from build123d import *

# Parameters (mm, degrees)
SKETCH2_R           = 2.55
SKETCH2_R_2         = 1.75
SKETCH2_R_3         = 11.5
SKETCH2_R_4         = 2.25
SKETCH2_R_5         = 2.6
BOSS_EXTRUDE1_DEPTH = 3


with BuildPart() as part:
    # Sketch2 → Boss-Extrude1 (new body)
    with BuildSketch(Plane(origin=(0, 0, 0), x_dir=(1, 0, 0), z_dir=(0, 1, 0))):
        with BuildLine():
            Line((0, -16.785), (0, 16.785))
            ThreePointArc((0, 16.785), (0.990365412, 21.123949711), (3.76529692, 24.603470279))
            Line((3.76529692, 24.603470279), (30.285548105, 45.751583128))
            ThreePointArc((30.285548105, 45.751583128), (42.973931455, 47.180980298), (49.767191801, 36.369418793))
            Line((49.767191801, 36.369418793), (49.767191801, 22.869418793))
            ThreePointArc((49.767191801, 22.869418793), (53.281910427, 14.384137419), (61.767191801, 10.869418793))
            Line((61.767191801, 10.869418793), (100.597191801, 10.869418793))
            ThreePointArc((100.597191801, 10.869418793), (105.807473987, 9.207876366), (109.093955082, 4.836743136))
            ThreePointArc((109.093955082, 4.836743136), (109.021446628, -3.277934075), (103.801176734, -9.490986945))
            Line((103.801176734, -9.490986945), (92.738459269, -15.929642261))
            ThreePointArc((92.738459269, -15.929642261), (89.099691246, -19.587512883), (87.768658735, -24.572390281))
            Line((87.768658735, -24.572390281), (87.768658735, -36.122390281))
            ThreePointArc((87.768658735, -36.122390281), (84.839726547, -43.193458093), (77.768658735, -46.122390281))
            Line((77.768658735, -46.122390281), (37.768658735, -46.122390281))
            ThreePointArc((37.768658735, -46.122390281), (34.279940347, -45.58043956), (31.120041688, -44.005667499))
            Line((31.120041688, -44.005667499), (4.218593872, -24.944371494))
            ThreePointArc((4.218593872, -24.944371494), (1.117037057, -21.377708281), (0, -16.785))
        make_face()
        with Locations(Location((37.767191801, 36.369418793, 0), (0, 0, 270))):
            Circle(SKETCH2_R, mode=Mode.SUBTRACT)
        with Locations(Location((37.767191801, 16.369418793, 0), (0, 0, 270))):
            Circle(SKETCH2_R_2, mode=Mode.SUBTRACT)
        with Locations(Location((22.26, 0.877609719, 0), (0, 0, 270))):
            Circle(SKETCH2_R_3, mode=Mode.SUBTRACT)
        with Locations(Location((37.767191801, -14.630581207, 0), (0, 0, 270))):
            Circle(SKETCH2_R_2, mode=Mode.SUBTRACT)
        with Locations(Location((6.767191801, -14.630581207, 0), (0, 0, 270))):
            Circle(SKETCH2_R_2, mode=Mode.SUBTRACT)
        with Locations(Location((6.767191801, 16.369418793, 0), (0, 0, 270))):
            Circle(SKETCH2_R_2, mode=Mode.SUBTRACT)
        with Locations(Location((52.26, 0.877609719, 0), (0, 0, 270))):
            Circle(SKETCH2_R_4, mode=Mode.SUBTRACT)
        with Locations(Location((78.26, 0.877609719, 0), (0, 0, 270))):
            Circle(SKETCH2_R_4, mode=Mode.SUBTRACT)
        with Locations(Location((97.86, 0.877609719, 0), (0, 0, 270))):
            Circle(SKETCH2_R_5, mode=Mode.SUBTRACT)
        with Locations(Location((37.767191801, -34.630581207, 0), (0, 0, 270))):
            Circle(SKETCH2_R, mode=Mode.SUBTRACT)
    extrude(amount=BOSS_EXTRUDE1_DEPTH)


solid = part.part
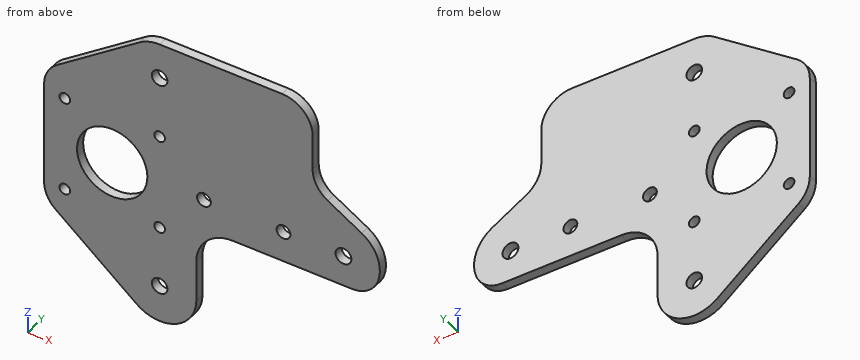
Verification items for the finished model (mm, model axes). Round coordinates to 2 decimals unless told otherwise and drop trailing zeros. Loops run counter-clockwise (first coordinate to the right, second up) from the corner with the lowest first, then second, coordinate; pieces in that order, holes last. Notation, with made-up numbers: (53.5, 2) - (90.5, 2) arc R18 cw to (90.5, 11) - close; hole circle Ø3 at (-36, 7). An arc over 180 degrees is marked (long way). Use a Markdown table: item, result. Add a question column.
1. Thickness scan on probe 1 along Z at (x, y) = (37.5, 1.7); probe 2 along X at (y, z) = (2.65, 0); probe 3 along X at (y, z) = (1.5, 0.5). Record the ranges inside material, lowest first. Write a range as [from, to].
2. Section check A-A, the plane x = 12. Record the boundary of the cut face in (y, z), plus the area to 3 significant figures.
3. Section check C-C, the plane x = 52.26. Record the boundary of the cut face in (y, z), plus the area to 3 significant figures.
4. Section check D-D, the plane x = 102.5. Record the boundary of the cut face in (y, z).
5. Section check B-B, the plane y = 1.7. Give the number of separate pieces and of enclosed holes in the cut face, plus the area to 3 significant figures.
6. Gauge pin test, flat ends, axial feed: pin 1 (5.5 mm diameter, centred on x = 6.77, z = -16.37, fed in from +Y); pin 2 (0.9 mm diameter, centred on y = 2, z = -31, fed in from +X); pin 3 (1 mm diameter, centred on y = 1, z = -36, fed in from -X); pin 4 (1.5 mm diameter, centred on y = 1.5, z = -36.5, fed in from -X). Record the tip position at first contact, or that the pin passes through.
Checks:
| question | item | result |
|---|---|---|
| 1 | probe 1 | z = [-48.37, -38.91], [-33.83, -18.1], [-14.64, 12.9], [16.36, 32.09], [37.17, 46.12] |
| 1 | probe 2 | x = [0, 10.79], [33.73, 50.19], [54.33, 76.19], [80.33, 95.41], [100.31, 109.73] |
| 1 | probe 3 | x = [0, 10.84], [33.68, 50.48], [54.04, 76.48], [80.04, 95.65], [100.07, 109.69] |
| 2 | outline | (0, -31.17) - (3, -31.17) - (3, -6.07) - (0, -6.07) - close; (0, 4.32) - (3, 4.32) - (3, 30.46) - (0, 30.46) - close |
| 2 | area | 154 mm^2 |
| 3 | outline | (0, -15.55) - (3, -15.55) - (3, -3.13) - (0, -3.13) - close; (0, 1.37) - (3, 1.37) - (3, 46.12) - (0, 46.12) - close |
| 3 | area | 172 mm^2 |
| 4 | outline | (0, -10.67) - (3, -10.67) - (3, 10.25) - (0, 10.25) - close |
| 5 | separate pieces | 1 |
| 5 | enclosed holes | 10 |
| 5 | area | 5,920 mm^2 |
| 6 | pin 1 | stops at y = 3 |
| 6 | pin 2 | stops at x = 49.77 |
| 6 | pin 3 | stops at x = 17.43 |
| 6 | pin 4 | stops at x = 17.74 |
